Autodesk Inventor part; units mm, degrees
ref_plane "РабПлоскость1" through (-4, 0, 0) normal (1, 0, 0) x (0, 0, -1)
ref_plane "YZ Plane" through (0, 0, 0) normal (1, 0, 0) x (0, 1, 0)
ref_plane "XZ Plane" through (0, 0, 0) normal (0, 1, 0) x (-1, 0, 0)
sketch "Эскиз1" plane through (0, 0, 0) normal (0, 1, 0) x (-1, 0, 0)
  circle A0 centre (0, 0) radius 1.4
  arc A1 (5.5622, -5.7499) -> (-8, 0) centre (0, 0) ccw
  line L0 (5.5622, -5.7499) -> (-4, -15)
  line L1 (-4, -15) -> (-8, -15)
  line L2 (-8, -15) -> (-8, 0)
  line L3 (-8, 0) -> (-8, 5.6017)
  line L4 (-8, 5.6017) -> (-2.7362, 7.5175)
  line L5 (-2.7362, 7.5175) -> (-8, 0)
  point P0 (-6, -15)
  dimension "d0" = 2.8
  dimension "d1" = 8
  dimension "d3" = 15
  dimension "d4" = 4
  dimension "d46" = 110
extrude "Выдавливание1" add sketch "Эскиз1" along normal blind 5 contours A0 | L0 L1 L2 L5 A1 | L5 A1 | A1 L3 L4
sketch "Эскиз2" plane through (0, 5, 0) normal (0, 1, 0) x (1, 0, 0)
  line L0 (-3.1754, 0) -> (-1.5877, 2.75)
  line L1 (-1.5877, 2.75) -> (1.5877, 2.75)
  line L2 (1.5877, 2.75) -> (3.1754, 0)
  line L3 (3.1754, 0) -> (1.5877, -2.75)
  line L4 (1.5877, -2.75) -> (-1.5877, -2.75)
  line L5 (-1.5877, -2.75) -> (-3.1754, 0)
  point P0 (0, 0)
  point P1 (0, 0)
  dimension "d8" = 5.5
extrude "Выдавливание2" cut sketch "Эскиз2" against normal blind 2
ref_plane "РабПлоскость1" through (-4, 0, 0) normal (1, 0, 0) x (0, 0, -1)
sketch "Эскиз5" plane through (8, 0, 0) normal (1, 0, 0) x (0, 0, -1)
  line L0 (5.7499, 5) -> (-8, 5)
  circle A0 centre (18, 30) radius 1.4
  arc A1 (20.5937, 28.4925) -> (15.4063, 31.5075) centre (18, 30) ccw
  line L1 (0, 5) -> (15.4063, 31.5075)
  line L2 (15, 0) -> (15, 5)
  line L3 (-5.6017, 5) -> (15, 5)
  line L4 (0, 5) -> (0, 3)
  line L5 (0, 5) -> (-8, 5)
  line L6 (-8, 0) -> (-8, 5)
  line L7 (-8, 0) -> (-8, 5)
  line L8 (5.7499, 0) -> (5.7499, 5)
  line L9 (-8, 0) -> (5.7499, 0)
  line L10 (6.9398, 5) -> (20.5937, 28.4925)
  line L11 (5.7499, 0) -> (6.9398, 5)
  point P0 (0, 0)
  dimension "d24" = 2.8
  dimension "d38" = 25
  dimension "d40" = 3
  dimension "d45" = 3
extrude "Выдавливание4" add sketch "Эскиз5" against normal blind 4 contours L0 L1 A1 L10 L3
sketch "Эскиз6" plane through (4, 0, 0) normal (-1, 0, 0) x (0, 0, 1)
  circle A0 centre (-18, 30) radius 1.4
  line L0 (-15, 0) -> (-15, 5)
  line L1 (-15, 0) -> (-13, 0)
  arc A1 (-13, 0) -> (-3.2532, 5) centre (-13, 12) ccw
  line L2 (-3.2532, 5) -> (-15, 5)
  line L3 (-15, 0) -> (-15, 28.4925)
  line L4 (-15, 0) -> (-15, 5)
  point P0 (0, 0)
  point P1 (-20.5937, 28.4925)
  point P2 (0, 5)
  dimension "d27" = 12
extrude "Выдавливание5" cut sketch "Эскиз6" along normal up to next contours L0 L2 A1 L1
chamfer "Фаска1" distance 1 angle 45 1 edges at (8, 30, -16.6)
sketch "Эскиз7" plane through (4, 0, 0) normal (-1, 0, 0) x (0, 0, 1)
  arc A0 (-15.4063, 31.5075) -> (-20.5937, 28.4925) centre (-18, 30) ccw
  circle A1 centre (-18, 30) radius 3
  circle A2 centre (-18, 30) radius 1.4
  point P0 (0, 0)
  dimension "d33" = 2.8
extrude "Выдавливание6" add sketch "Эскиз7" along normal blind 2
sketch "Эскиз10" plane through (8, 0, 0) normal (1, 0, 0) x (0, 0, -1)
  line L0 (6.9398, 5) -> (20.5937, 28.4925)
  line L1 (6.9398, 5) -> (6.9398, 0)
  line L2 (0, 0) -> (15, 0)
  line L3 (6.9398, 5) -> (15, 5)
  line L4 (6.9398, 5) -> (15, 5)
  line L5 (15, 5) -> (15, 0)
extrude "Выдавливание7" cut sketch "Эскиз10" against normal up to next
sketch "Эскиз11" plane through (2, 30, -18) normal (-1, 0, 0) x (0, 0, 1)
  point P0 (18, -30)
fillet "Сопряжение1" radius 9 1 edges at (6, 5, -6.9398)
sketch "Эскиз12" plane through (0, 3, 0) normal (0, 1, 0) x (1, 0, 0)
  point P0 (0, 0)
  point P1 (0, 0)
hole "Отверстие1" at (0, 3, 0) direction (0, -1, 0) diameter 3 end through all
properties part number "Wheelholder" material "Пластик АБС"
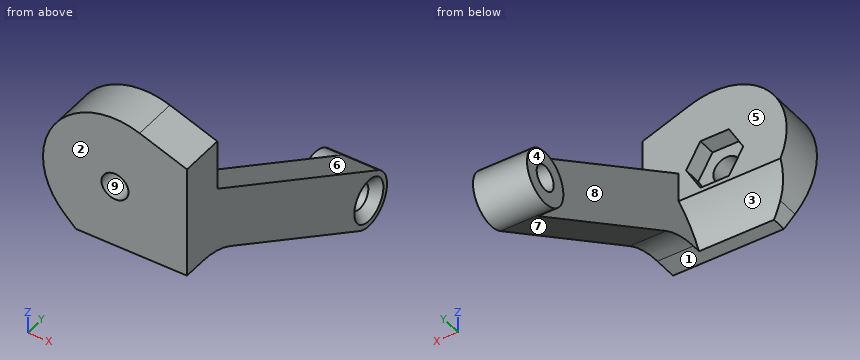
Work out the finished part from the listing and answer in its coordinate system (mm). Face numbers are marked on the shaded views. A direction names the side the tool comes from. Coordinates: 2 decimals unless noted, no trailing zeros. Write each loop counter-clockwise with the first axis right and the second up, starting at its lowest first coordinate (ties: lowest second). Pieces come first, ordered by that corner, then holes. Notation, with made-up numbers: (36.5, 46.25) - (71.5, 46.25) arc R29 ccw to (71.5, 69.25) - close; hole circle Ø11 at (28.5, 41.25). An arc over 180 degrees is marked (long way). One line per question, with ' | ' between items.
1) The mould has two halves that part along Z. Classify the marked faces 6, 7, 8 and 9: +Z half, -Z half, draft (parallel to the pull), parting line (faces both ways), or undercut.
Checks:
face 6: +Z half | face 7: -Z half | face 8: draft | face 9: undercut
2) For the marked faces 1, 2, 3, 4 and 5, determine the directions among +Z, -Z, +X, -X, +Y, -Y from which every point of the face is accessible in a straight line to the end or side of a thin tool.
Checks:
face 1: -Z, +X, -X, -Y | face 2: +Z, -Z, +X, -X, -Y | face 3: -Z, -X, +Y | face 4: +Z, -Z, -X, +Y, -Y | face 5: +Z, -X, +Y
3) Find section B-B, the plane x = 4.5. Determine the outline of the cut face in (y, z), and give its area (3 significant figures).
Checks:
outline: (0, -6.94) - (2.57, -6.94) arc R9 cw to (7.1, -8.16) - (28.49, -20.59) arc R3 ccw to (31.51, -15.41) - (5, 0) - (5, 6.88) - (0, 6.88) - close; hole circle Ø2.8 at (30, -18) | area: 251 mm2
4) Consider probe 1 along X at (y, z) = (2.3, 0); probe 2 along Z at (x, y) = (0, 1.4); probe 3 along Y at (x, z) = (3.8, -18). Determine where each line is inside the solid, lowest interval first. Write a range as [from, to].
Checks:
probe 1: [-8, -1.5], [1.5, 8] | probe 2: [-6.94, -1.5], [1.5, 8] | probe 3: [27, 28.6], [31.4, 33]
5) Find section C-C, the plane y = 30. Determine the outline of the cut face in (x, z).
Checks:
outline: (2, -21) - (8, -21) - (8, -20.4) - (7, -19.4) - (2, -19.4) - close; (2, -16.6) - (7, -16.6) - (8, -15.6) - (8, -14.53) - (4, -14.53) - (4, -15) - (2, -15) - close
6) Flat-ended cylindrical pins translate along their axes: P1, Ø3, axis at x = 4.5, y = 10.5, coming from the +Z side; P2, Ø5, axis at x = 5.5, z = -11.5, coming from the +Y side; P3, Ø4, axis at x = 2.5, z = 3.5, coming from the +Y side. Find the tip coordinate at first contact, or state that the pin passes through.
Checks:
P1: z = -2.32 | P2: y = 29.09 | P3: y = 5
7) Find section A-A, the plane x = 0. Determine the outline of the cut face in (y, z), and give its area (3 significant figures).
Checks:
outline: (0, -6.94) - (1.64, -6.94) arc R12 cw to (5, -3.25) - (5, -2.75) - (3, -2.75) - (3, -1.5) - (0, -1.5) - close; (0, 1.5) - (3, 1.5) - (3, 2.75) - (5, 2.75) - (5, 8) - (0, 8) - close | area: 47.6 mm2
8) Find section D-D, the plane y = 4. Determine the outline of the cut face in (x, z).
Checks:
outline: (-6.9, -4.06) - (4, -4.06) - (4, -7.05) - (8, -7.05) - (8, 5.6) - (2.74, 7.52) arc R8 ccw to start; hole (-3.18, 0) - (-1.59, -2.75) - (1.59, -2.75) - (3.18, 0) - (1.59, 2.75) - (-1.59, 2.75) - close
